Autodesk Inventor part; units mm, degrees
ref_plane "YZ Plane" through (0, 0, 0) normal (1, 0, 0) x (0, 1, 0)
ref_plane "XZ Plane" through (0, 0, 0) normal (0, 1, 0) x (-1, 0, 0)
ref_plane "XY Plane" through (0, 0, 0) normal (0, 0, 1) x (1, 0, 0)
sketch "Sketch1" plane through (0, 0, 0) normal (0, 1, 0) x (-1, 0, 0)
  circle A0 centre (0, 0) radius 15
  dimension "d0" = 30
extrude "Extrusion1" add sketch "Sketch1" along normal blind 9
sketch "Sketch3" plane through (0, 9, 0) normal (0, 1, 0) x (1, 0, 0)
  circle A0 centre (0, 0) radius 11 construction
  line L0 (0, 0) -> (0, 11) construction
  line L1 (0, 11) -> (7.7782, 7.7782) construction
  line L2 (7.7782, 7.7782) -> (11, 0) construction
  line L3 (11, 0) -> (7.7782, -7.7782) construction
  line L4 (7.7782, -7.7782) -> (0, -11) construction
  line L5 (0, -11) -> (-7.7782, -7.7782) construction
  line L6 (-7.7782, -7.7782) -> (-11, 0) construction
  line L7 (-11, 0) -> (-7.7782, 7.7782) construction
  line L8 (-7.7782, 7.7782) -> (0, 11) construction
  circle A1 centre (-11, 0) radius 1.4
  circle A2 centre (-7.7782, 7.7782) radius 1.4
  circle A3 centre (-7.7782, -7.7782) radius 1.4
  circle A4 centre (0, -11) radius 1.4
  circle A5 centre (7.7782, -7.7782) radius 1.4
  circle A6 centre (11, 0) radius 1.4
  circle A7 centre (7.7782, 7.7782) radius 1.4
  circle A8 centre (0, 11) radius 1.4
  dimension "d12" = 22
  dimension "d13" = 2.8
  dimension "d14" = 2.8
  dimension "d15" = 2.8
  dimension "d16" = 2.8
  dimension "d17" = 2.8
  dimension "d18" = 2.8
  dimension "d19" = 2.8
  dimension "d20" = 2.8
extrude "Extrusion3" cut sketch "Sketch3" against normal up to next
sketch "Sketch4" plane through (0, 9, 0) normal (0, 1, 0) x (1, 0, 0)
  circle A0 centre (-11, 0) radius 1.4 construction
  circle A1 centre (0, 0) radius 11 construction
  line L0 (0, 0) -> (-11, 0) construction
  line L1 (-11, 0) -> (-7.7782, 7.7782) construction
  line L2 (-7.7782, 7.7782) -> (0, 11) construction
  line L3 (0, 11) -> (7.7782, 7.7782) construction
  line L4 (7.7782, 7.7782) -> (11, 0) construction
  line L5 (11, 0) -> (7.7782, -7.7782) construction
  line L6 (7.7782, -7.7782) -> (0, -11) construction
  line L7 (0, -11) -> (-7.7782, -7.7782) construction
  line L8 (-7.7782, -7.7782) -> (-11, 0) construction
  circle A2 centre (-11, 0) radius 2.6
  circle A3 centre (-7.7782, 7.7782) radius 1.4
  circle A4 centre (-7.7782, 7.7782) radius 2.6
  circle A5 centre (0, 11) radius 2.6
  circle A6 centre (7.7782, 7.7782) radius 2.6
  circle A7 centre (11, 0) radius 2.6
  circle A8 centre (7.7782, -7.7782) radius 1.4
  circle A9 centre (7.7782, -7.7782) radius 2.6
  circle A10 centre (0, -11) radius 1.4
  circle A11 centre (0, -11) radius 2.6
  circle A12 centre (-7.7782, -7.7782) radius 2.6
  dimension "d23" = 5.2
  dimension "d24" = 5.2
  dimension "d25" = 5.2
  dimension "d26" = 5.2
  dimension "d27" = 5.2
  dimension "d28" = 5.2
  dimension "d29" = 5.2
  dimension "d30" = 5.2
extrude "Extrusion4" cut sketch "Sketch4" against normal blind 3.5
sketch "Sketch5" plane through (0, 0, 0) normal (0, -1, 0) x (1, 0, 0)
  circle A0 centre (0, 0) radius 6
  dimension "d33" = 12
extrude "Extrusion5" cut sketch "Sketch5" against normal blind 7
sketch "Skizze6" plane through (0, 9, 0) normal (0, 1, 0) x (1, 0, 0)
  circle A0 centre (0, 0) radius 6
  circle A1 centre (0, 0) radius 5
  dimension "d36" = 10
extrude "Extrusion6" add sketch "Skizze6" along normal blind 35 contours A1
properties part number "motorhorn_zu_ftsensor"
The model under review builds one solid part; all positions refer to its coordinate system, in mm. A direction names the side the tool comes from. Round coordinates to 2 decimals unless told otherwise and drop trailing zeros. Write each loop counter-clockwise with the first axis right and the second up, starting at its lowest first coordinate (ties: lowest second). Pieces come first, ordered by that corner, then holes. Notation, with made-up numbers: (47.25, 25) -> (64.25, 25) arc R38 ccw to (64.25, 64) -> close; hole circle Ø11 at (27.5, 64). An arc over 180 degrees is marked (long way). Answer as a JSON object with one key per item and string values.
1. We need section D-D on x = -11. State the section outline as (y, z) points, and give its area (3 significant figures).
Results found:
{"outline": "(0, -10.2) -> (9, -10.2) -> (9, -2.6) -> (5.5, -2.6) -> (5.5, -1.4) -> (0, -1.4) -> close; (0, 1.4) -> (5.5, 1.4) -> (5.5, 2.6) -> (9, 2.6) -> (9, 10.2) -> (0, 10.2) -> close", "area": "150 mm^2"}
2. We need section A-A on z = 0. State the section outline as (x, y) points, and give its area (3 significant figures).
Results found:
{"outline": "(-15, 0) -> (-12.4, 0) -> (-12.4, 5.5) -> (-13.6, 5.5) -> (-13.6, 9) -> (-15, 9) -> close; (-9.6, 0) -> (-6, 0) -> (-6, 7) -> (6, 7) -> (6, 0) -> (9.6, 0) -> (9.6, 5.5) -> (8.4, 5.5) -> (8.4, 9) -> (5, 9) -> (5, 44) -> (-5, 44) -> (-5, 9) -> (-8.4, 9) -> (-8.4, 5.5) -> (-9.6, 5.5) -> close; (12.4, 0) -> (15, 0) -> (15, 9) -> (13.6, 9) -> (13.6, 5.5) -> (12.4, 5.5) -> close", "area": "469 mm^2"}
3. To check wall thickness, follow line 1 along Z through (x, y) = (0, 1.9); line 2 along Z through (x, y) = (0, 6.6); line 3 along Y through (x, z) = (9, -6.75). State the ranges of each line that lie inside material, in increasing order.
Results found:
{"line 1": "z = -15 to -12.4, -9.6 to -6, 6 to 9.6, 12.4 to 15", "line 2": "z = -15 to -13.6, -8.4 to -6, 6 to 8.4, 13.6 to 15", "line 3": "y = 0 to 5.5"}
4. Machinability: for faces 1 (the face through (-9.9, 5.5, 1.1)), 2 (the face through (0.75, 2.79, 9.82)), which of the approach directions +Z, -Z, +X, -X, +Y, -Y give a long, thin tool a straight path to every point of the face, cutting with its end or side? Answer none if there is none.
Results found:
{"face 1": "+Y", "face 2": "+Y, -Y"}
5. Clearance check with flat-ended pins moving along their axes: pin 1 (3 mm diameter, centred on y = 19.5, z = -2, fed in from +X); pin 2 (12 mm diameter, centred on x = -7.5, y = 36.5, fed in from -Z); pin 3 (4 mm diameter, centred on x = -0.5, z = -10.5, fed in from +Y). State where each tip first meets the part, or that it passes through.
Results found:
{"pin 1": "stops at x = 4.97", "pin 2": "stops at z = -4.77", "pin 3": "stops at y = 9"}
6. We need section C-C on z = 11. State the section outline as (x, y) points.
Results found:
{"outline": "(-10.2, 0) -> (-1.4, 0) -> (-1.4, 5.5) -> (-2.6, 5.5) -> (-2.6, 9) -> (-10.2, 9) -> close; (1.4, 0) -> (10.2, 0) -> (10.2, 9) -> (2.6, 9) -> (2.6, 5.5) -> (1.4, 5.5) -> close"}
7. We need section B-B on x = -0.25. State the section outline as (y, z) points.
Results found:
{"outline": "(0, -15) -> (9, -15) -> (9, -13.59) -> (5.5, -13.59) -> (5.5, -12.38) -> (0, -12.38) -> close; (0, -9.62) -> (5.5, -9.62) -> (5.5, -8.41) -> (9, -8.41) -> (9, -4.99) -> (44, -4.99) -> (44, 4.99) -> (9, 4.99) -> (9, 8.41) -> (5.5, 8.41) -> (5.5, 9.62) -> (0, 9.62) -> (0, 5.99) -> (7, 5.99) -> (7, -5.99) -> (0, -5.99) -> close; (0, 12.38) -> (5.5, 12.38) -> (5.5, 13.59) -> (9, 13.59) -> (9, 15) -> (0, 15) -> close"}
